Work out the finished part from the listing and answer in its coordinate system (mm). A direction names the side the tool comes from. Coordinates: 2 decimals unless noted, no trailing zeros. Write each loop counter-clockwise with the first axis right and the second up, starting at its lowest first coordinate (ties: lowest second). Pieces come first, ordered by that corner, then holes. Notation, with made-up numbers: M 1.25,30.5 L 17.25,30.5 A25 ccw 17.25,64.5 Z; hole C -21.5,86.25 d5. An arc over 180 degrees is marked long. Answer as CSV lines item,"result". Start each with the question number.
(1) The mould has two halves that part along X. Classify faces 4 (the conical face through (-5.96, 12.63, 12.48)), 5 (the flat face through (-0.745, 11.847, 1.24)), 6 (the flat face through (0, 0, -1)): released by +X, released by -X, zero draft, split by the parting line, or undercut.
(2) A cutting plane is placed at C-C on x = -6. Give the vertices of the cut face in (y, z), then the cut area to 3 significant figures.
(3) Find the intervals of material crossed by L1, parallel to X at y = 13.5, z = 8 (3 decimals); L2, parallel to Y at x = -8.5, z = 9.5; L3, parallel to Z at x = -2, y = 3.5, in increasing order. Write a range as [from, to].
(4) For faces 1 (the flat face through (-8.8, 10, 11)), 2 (the cylindrical face through (-9.94, 10.41, 10.25)), 3 (the cylindrical face through (2.403, -1.962, 7.449)), determine the directions among +Z, -Z, +X, -X, +Y, -Y from which every point of the face is accessible in a straight line to the end or side of a thin tool.
(5) A cutting plane is placed at A-A on z = -3.75. Give the vertices of the cut face in (x, y).
(6) Flat-ended cylindrical pins translate along their axes: P1, Ø17, axis at y = -2.5, z = -4, coming from the -X side; P2, Ø8, axis at x = -7, z = 11, coming from the -Y side; P3, Ø5, axis at x = -8, y = 15, coming from the +Z side; P4, Ø1.5, axis at x = -8.5, y = 1, coming from the -Z side. Find the tip coordinate at first contact, or state that the pin passes through.
(7) A cutting plane is placed at D-D on x = -9.75. Give the vertices of the cut face in (y, z), then the cut area to 3 significant figures.
(8) A cutting plane is placed at B-B on y = -0.5. Give the vertices of the cut face in (x, z).
from build123d import *

# Parameters (mm, degrees)
F1_ANGLE = 90
F3_DEPTH = 10
F4_DEPTH = 10
F6_DEPTH = 25


with BuildPart() as f1:
    # F0 (on Top) → F1 (revolve)
    with BuildSketch(Plane.XY):
        with BuildLine():
            Line((0, 5.4679050659), (0, 0))
            Line((0, 0), (2.5, 0))
            Line((2.5, 0), (2.5, 5.4679050659))
            ThreePointArc((2.5, 5.4679050659), (0.9585130135, 13.202552711), (-3.4303982666, 19.7552936717))
            Line((-3.4303982666, 19.7552936717), (-8.4106450471, 20.863986155))
            Line((-8.4106450471, 20.863986155), (-10.1253781611, 18.1776133961))
            ThreePointArc((-10.1253781611, 18.1776133961), (-10.8847896659, 16.4666549044), (-11.1032370478, 14.6075245875))
            Line((-11.1032370478, 14.6075245875), (-8.8, 14.6075245875))
            Line((-8.8, 14.6075245875), (-8.8, 15.6075245875))
            Line((-8.8, 15.6075245875), (-7.2452009387, 18.0433379567))
            Line((-7.2452009387, 18.0433379567), (-4.7073274561, 17.4783616859))
            ThreePointArc((-4.7073274561, 17.4783616859), (-1.2188561035, 11.9179050659), (0, 5.4679050659))
        make_face()
    revolve(axis=Axis((1.25, 0, 0), (1, 0, 0)), revolution_arc=F1_ANGLE)

    # F3 (add): a face of the model
    f3_faces = [f1.faces().sort_by_distance(p)[0] for p in [
        (-0.9869443197, 12.0087995874, 0),
    ]]
    extrude(f3_faces, amount=F3_DEPTH)

    # F4 (add): a face of the model
    f4_faces = [f1.faces().sort_by_distance(p)[0] for p in [
        (-0.9048130801, 0, 12.0409897573),
    ]]
    extrude(f4_faces, amount=F4_DEPTH)

    # F5 (on face) → F6 (intersect)
    with BuildSketch(Plane.YZ.offset(2.5)):
        Polygon((12.4376601817, 23.0442618995), (-10, 0.6066017178), (0.6066017178, -10), (23.0442618995, 12.4376601817), align=None)
    extrude(amount=-F6_DEPTH, mode=Mode.INTERSECT)


solid = f1.part
Here are the results:
1,face 4,"undercut"
1,face 5,"zero draft"
1,face 6,"released by -X"
2,outline,"M 6.08,16.69 A17.77 cw 16.69,6.08 L 18.66,8.06 A20.33 ccw 8.06,18.66 Z"
2,area,"39.5 mm^2"
3,L1,"x = [-11.045, -8.746], [-3.257, -0.283]"
3,L2,"y = [12.97, 18.42]"
3,L3,"z = [13.18, 14.11]"
4,face 1,"-Z, -Y"
4,face 2,"-Z, -X, -Y"
4,face 3,"+Z, +X, +Y, -Y"
5,outline,"M -0.05,6.86 A17.68 cw 0,5.47 L 0,-5.64 L 2.5,-5.64 L 2.5,5.47 A20.18 ccw 2.45,6.86 Z"
6,P1,"stops at x = -0.01"
6,P2,"stops at y = 3.56"
6,P3,"stops at z = 16.68"
6,P4,"passes through"
7,outline,"M 3.56,14.17 A14.61 cw 14.17,3.56 L 17.47,6.86 A18.77 ccw 6.86,17.47 Z"
7,area,"64.7 mm^2"
8,outline,"M -0.62,10.11 A17.68 cw 0,5.47 L 0,-8.89 L 2.5,-8.89 L 2.5,5.47 A20.18 ccw 1.96,10.11 Z"
